Can you work these out from the model? Positions are in its coordinate system, mm. A direction names the side the tool comes from. Round coordinates to 2 decimals unless told otherwise and drop trailing zeros. Write each loop counter-clockwise with the first axis right and the second up, starting at its lowest first coordinate (ties: lowest second). Pieces come first, ordered by that corner, then holes. Notation, with made-up numbers: (-3.5, 48.5) -> (11.5, 48.5) arc R6 cw to (11.5, 55.5) -> close; hole circle Ø1 at (46.25, 21). An arc over 180 degrees is marked (long way). Write item = value, one per line. Start each with the question number.
1) If I drill on line 1 (Z direction, x = -6, y = 0.2); line 2 (X direction, y = 1.2, z = 14.94); line 3 (X direction, y = 1.1, z = -19), over which ranges is the centre line in solid material (lowest first)?
2) For faces 5 (the face through (0, 1, -28.5)), 6 (the face through (56.65, 1.01, 30.64)), which set-ups out of +Z, -Z, +X, -X, +Y, -Y let a thin tool reach every point of the face, with its end or its side?
3) Imagine slicing it at A-A, the plane z = -19. Please give me the cut outline in (x, y).
4) Imagine slicing it at C-C, the plane y = 1.55. State how many separate pieces and enclosed holes the cut face has, then the cut area to 3 significant figures.
5) Imagine slicing it at B-B, the plane x = 3.5. Please give me the cut outline in (y, z), then the cut area to 3 significant figures.
6) I'm going to push flat-ended pins straight in: pin 1 (3.5 mm diameter, centred on x = -22.09, z = -14.94, fed in from -Y); pin 2 (2.5 mm diameter, centred on x = 53.55, z = -27.5, fed in from -Y). Where does each tip first touch, or does it pass through?
7) Thinking about a two-plate mould opening in X: for faces 1 (the face through (-51.774, 1.014, -28.423)), 2 (the face through (-1, 1, -31.5)), 3 (the face through (-56.69, 1.01, -30.6)), 4 (the face through (51.774, 1.014, -26.577)), which applies, +X half, -X half, draft (parallel to the pull), parting line (faces both ways), or undercut?
from build123d import *

# Parameters (mm, degrees)
ESBO_O1_W                = 115.09677689
ESBO_O1_H                = 63
RESSALTO_EXTRUS_O1_DEPTH = 2
ESBO_O2_R                = 1.55
CORTE_EXTRUS_O1_DEPTH    = 66.635866816
ESBO_O3_W                = 18
ESBO_O3_H                = 6
CORTE_EXTRUS_O2_DEPTH    = 66.635866816
ESBO_O5_R                = 2
CORTE_EXTRUS_O3_DEPTH    = 66.635866816
FILETE1_R                = 3
ESBO_O8_R                = 1.2
CORTE_EXTRUS_O4_DEPTH    = 66.635866816


with BuildPart() as part:
    # Esboço1 → Ressalto-extrusão1 (new body)
    with BuildSketch(Plane(origin=(0, 0, 0), x_dir=(1, 0, 0), z_dir=(0, 1, 0))):
        Rectangle(ESBO_O1_W, ESBO_O1_H)
    extrude(amount=RESSALTO_EXTRUS_O1_DEPTH)

    # Esboço2 → Corte-extrusão1 (cut, through all)
    with BuildSketch(Plane(origin=(0, 2, 0), x_dir=(1, 0, 0), z_dir=(0, 1, 0))):
        with Locations(Location((-46.153556516, -14.945, 0), (0, 0, 270))):
            Circle(ESBO_O2_R)
        with Locations(Location((-22.093556516, -14.94, 0), (0, 0, 270))):
            Circle(ESBO_O2_R)
        with Locations(Location((22.093556516, -14.94, 0), (0, 0, 90))):
            Circle(ESBO_O2_R)
        with Locations(Location((46.153556516, -14.945, 0), (0, 0, 90))):
            Circle(ESBO_O2_R)
        with Locations(Location((46.153556516, 14.945, 0), (0, 0, 270))):
            Circle(ESBO_O2_R)
        with Locations(Location((22.093556516, 14.94, 0), (0, 0, 270))):
            Circle(ESBO_O2_R)
        with Locations(Location((-22.093556516, 14.94, 0), (0, 0, 90))):
            Circle(ESBO_O2_R)
        with Locations(Location((-46.153556516, 14.945, 0), (0, 0, 90))):
            Circle(ESBO_O2_R)
    extrude(amount=-CORTE_EXTRUS_O1_DEPTH, mode=Mode.SUBTRACT)

    # Esboço3 → Corte-extrusão2 (cut, through all)
    with BuildSketch(Plane.XZ):
        with Locations((0, 25.5)):
            Rectangle(ESBO_O3_W, ESBO_O3_H)
        with Locations((0, -25.5)):
            Rectangle(ESBO_O3_W, ESBO_O3_H)
    extrude(amount=-CORTE_EXTRUS_O2_DEPTH, mode=Mode.SUBTRACT)

    # Esboço5 → Corte-extrusão3 (cut, through all)
    with BuildSketch(Plane(origin=(0, 2, 0), x_dir=(1, 0, 0), z_dir=(0, 1, 0))):
        with Locations(Location((53.548388445, 27.5, 0), (0, 0, 270))):
            Circle(ESBO_O5_R)
        with Locations(Location((53.548388445, -27.5, 0), (0, 0, 90))):
            Circle(ESBO_O5_R)
        with Locations(Location((-53.548388445, -27.5, 0), (0, 0, 270))):
            Circle(ESBO_O5_R)
        with Locations(Location((-53.548388445, 27.5, 0), (0, 0, 90))):
            Circle(ESBO_O5_R)
    extrude(amount=-CORTE_EXTRUS_O3_DEPTH, mode=Mode.SUBTRACT)

    # Filete1
    filete1_edges = [part.edges().sort_by_distance(p)[0] for p in [
        (-57.548388445, 1, -31.5),
        (57.548388445, 1, -31.5),
        (57.548388445, 1, 31.5),
        (-57.548388445, 1, 31.5),
    ]]
    fillet(filete1_edges, radius=FILETE1_R)

    # Esboço8 → Corte-extrusão4 (cut, through all)
    with BuildSketch(Plane(origin=(0, 2, 0), x_dir=(1, 0, 0), z_dir=(0, 1, 0))):
        with Locations(Location((-12.498388445, 28.5, 0), (0, 0, 270))):
            Circle(ESBO_O8_R)
        with Locations(Location((12.498388445, 28.5, 0), (0, 0, 90))):
            Circle(ESBO_O8_R)
        with Locations(Location((12.498388445, -28.5, 0), (0, 0, 270))):
            Circle(ESBO_O8_R)
        with Locations(Location((-12.498388445, -28.5, 0), (0, 0, 90))):
            Circle(ESBO_O8_R)
        with Locations(Location((-8.998388445, -19, 0), (0, 0, 270))):
            Circle(ESBO_O8_R)
        with Locations(Location((8.998388445, -19, 0), (0, 0, 90))):
            Circle(ESBO_O8_R)
        with Locations(Location((8.998388445, 19, 0), (0, 0, 270))):
            Circle(ESBO_O8_R)
        with Locations(Location((-8.998388445, 19, 0), (0, 0, 90))):
            Circle(ESBO_O8_R)
    extrude(amount=-CORTE_EXTRUS_O4_DEPTH, mode=Mode.SUBTRACT)


solid = part.part
Reported:
q1.line_1 = -31.5 to -28.5, -22.5 to 22.5, 28.5 to 31.5
q1.line_2 = -57.55 to -47.7, -44.6 to -23.64, -20.54 to 20.54, 23.64 to 44.6, 47.7 to 57.55
q1.line_3 = -57.55 to -10.2, -7.8 to 7.8, 10.2 to 57.55
q2.face_5 = +Y, -Y
q2.face_6 = +Z, +X, +Y, -Y
q3.outline = (-57.55, 0) -> (-10.2, 0) -> (-10.2, 2) -> (-57.55, 2) -> close; (-7.8, 0) -> (7.8, 0) -> (7.8, 2) -> (-7.8, 2) -> close; (10.2, 0) -> (57.55, 0) -> (57.55, 2) -> (10.2, 2) -> close
q4.separate_pieces = 1
q4.enclosed_holes = 22
q4.area = 6,880 mm²
q5.outline = (0, -31.5) -> (2, -31.5) -> (2, -28.5) -> (0, -28.5) -> close; (0, -22.5) -> (2, -22.5) -> (2, 22.5) -> (0, 22.5) -> close; (0, 28.5) -> (2, 28.5) -> (2, 31.5) -> (0, 31.5) -> close
q5.area = 102 mm²
q6.pin_1 = 0
q6.pin_2 = through
q7.face_1 = undercut
q7.face_2 = draft
q7.face_3 = -X half
q7.face_4 = undercut
